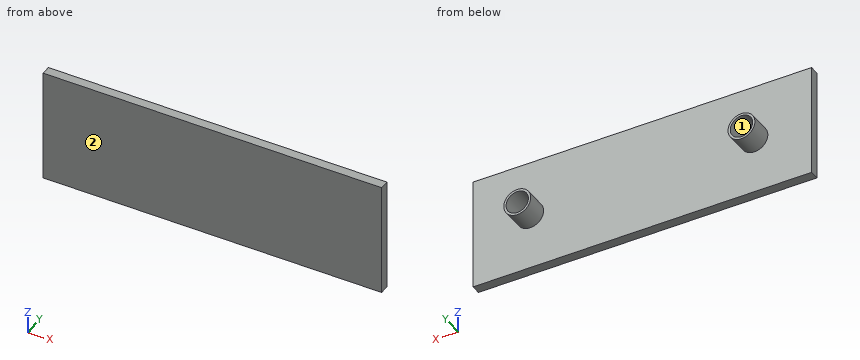
from build123d import *

# Parameters (mm, degrees)
SKETCH1_W               = 75.5
SKETCH1_H               = 25
BOSS_EXTRUDE1_DEPTH     = 2.1
CUT_EXTRUDE1_DEPTH      = 0.2
CUT_EXTRUDE1_DEPTH_BACK = 0.2
SKETCH4_R               = 3
SKETCH4_R_2             = 2.5
BOSS_EXTRUDE2_DEPTH     = 5
SKETCH5_R               = 2.5
CUT_EXTRUDE5_DEPTH      = 0.5


with BuildPart() as part:
    # Sketch1 → Boss-Extrude1 (new body)
    with BuildSketch(Plane(origin=(0, 0, 0), x_dir=(1, 0, 0), z_dir=(0, 1, 0))):
        with Locations((-9.096373467, 8.083487785)):
            Rectangle(SKETCH1_W, SKETCH1_H)
    extrude(amount=BOSS_EXTRUDE1_DEPTH)

    # Sketch3 → Cut-Extrude1 (cut, two sides)
    with BuildSketch(Plane(origin=(0, 1.05, 0), x_dir=(-1, 0, 0), z_dir=(0, -1, 0))) as cut_extrude1_sk:
        with BuildLine():
            Line((34.096373467, 5.583487785), (-15.903626533, 5.583487785))
            ThreePointArc((-15.903626533, 5.583487785), (-18.403626533, 8.083487785), (-15.903626533, 10.583487785))
            Line((-15.903626533, 10.583487785), (34.096373467, 10.583487785))
            ThreePointArc((34.096373467, 10.583487785), (36.596373467, 8.083487785), (34.096373467, 5.583487785))
        make_face()
    extrude(amount=CUT_EXTRUDE1_DEPTH, mode=Mode.SUBTRACT)
    extrude(cut_extrude1_sk.sketch, amount=-CUT_EXTRUDE1_DEPTH_BACK, mode=Mode.SUBTRACT)

    # Sketch4 → Boss-Extrude2 (add)
    with BuildSketch(Plane(origin=(0, 2.1, 0), x_dir=(1, 0, 0), z_dir=(0, 1, 0))):
        with Locations((-34.096373467, 8.083487785)):
            Circle(SKETCH4_R)
        with Locations((-34.096373467, 8.083487785)):
            Circle(SKETCH4_R_2, mode=Mode.SUBTRACT)
        with Locations((15.903626533, 8.083487785)):
            Circle(SKETCH4_R)
        with Locations((15.903626533, 8.083487785)):
            Circle(SKETCH4_R_2, mode=Mode.SUBTRACT)
    extrude(amount=BOSS_EXTRUDE2_DEPTH)

    # Sketch5 → Cut-Extrude5 (cut)
    with BuildSketch(Plane.XZ.offset(-1.25)):
        with Locations((-34.096373467, -8.083487785)):
            Circle(SKETCH5_R)
        with Locations((15.903626533, -8.083487785)):
            Circle(SKETCH5_R)
    extrude(amount=-CUT_EXTRUDE5_DEPTH, mode=Mode.SUBTRACT)


solid = part.part
Could you check a few things on this model? Use its own coordinates, in mm. Face numbers are marked on the shaded views. Coordinates: 2 decimals unless noted, no trailing zeros. Write each loop counter-clockwise with the first axis right and the second up, starting at its lowest first coordinate (ties: lowest second). Pieces come first, ordered by that corner, then holes. Notation, with made-up numbers: (81.25, 72) - (86.25, 72) arc R22 ccw to (86.25, 104) - close; hole circle Ø4 at (-35, 34.25). An arc over 180 degrees is marked (long way). Put each result on its own line as item: value. Start each with the question number.
Q1. I want a section at D-D on x = 20.5. Write out the boundary of the cut face in (y, z).
Q2. I want a section at C-C on z = -18.5. Write out the boundary of the cut face in (x, y), plus the area to 3 significant figures.
Q3. I'm going to push a flat-ended pin straight in: P1, Ø4, axis at x = -34.1, z = -8.08, coming from the +Y side. Where does the tip first touch, or does it pass through?
Q4. I want a section at B-B on y = 6. Write out the boundary of the cut face in (x, z).
Q5. I want a section at A-A on x = -1. Write out the boundary of the cut face in (y, z).
Q6. Thinking about a two-plate mould opening in X: for the marked faces 1 and 2, which applies, pulls with the +X half, pulls with the -X half, needs draft (parallel to the pull), parting line crosses it, or undercut?
Q7. Please list where these lines run through material, in increasing order: L1, parallel to Y at x = -19, z = -9.75; L2, parallel to X at y = 4.75, z = -6.25; L3, parallel to Y at x = -20, z = 2.5.
Checks:
1. outline: (0, -20.58) - (2.1, -20.58) - (2.1, 4.42) - (0, 4.42) - close
2. outline: (-46.85, 0) - (28.65, 0) - (28.65, 2.1) - (-46.85, 2.1) - close
2. area: 159 mm²
3. P1: y = 2.1
4. outline: circle Ø6 at (-34.1, -8.08); circle Ø6 at (15.9, -8.08); hole circle Ø5 at (-34.1, -8.08); hole circle Ø5 at (15.9, -8.08)
5. outline: (0, -20.58) - (2.1, -20.58) - (2.1, 4.42) - (0, 4.42) - close; hole (0.85, -10.58) - (1.25, -10.58) - (1.25, -5.58) - (0.85, -5.58) - close
6. face 1: undercut
6. face 2: needs draft
7. L1: 0 to 0.85, 1.25 to 2.1
7. L2: -36.47 to -35.8, -32.4 to -31.72, 13.53 to 14.2, 17.6 to 18.28
7. L3: 0 to 2.1
